Answer from the drawing. Dimensions are ordinates in mm from the lowest x, y and z of the part. Coordinates: 2 decimals unless noted, no trailing zeros. Order: outer loops, then holes, each group sorted by start corner. A loop starts at its lowest first (then second) coordinate and runs counter-clockwise, first axis right, second up. Notation, with made-up numbers: (44.5, -7.5) - (91.5, -7.5) arc R19 ccw to (91.5, -3.5) - close; hole circle Ø4 at (-14, 71). An arc over 180 degrees is marked (long way). Answer as a JSON object with one key per item and string values. Group by question number.
1) Section A-A (x = 45) is taken. Give the vertices of the cut face in (y, z), plus the area to 3 significant figures.
2) Each of these flat-tipped pins is pushed along its axis until it touches: P1, Ø5, axis at x = 49, y = 64.5, coming from the +Z side; P2, Ø4, axis at x = 49, z = 29.5, coming from the +Y side; P3, Ø5, axis at x = 15, z = 20, coming from the +Y side. Where does it stop, or does it pass through?
3) The mould has two halves that part along X. Classify the marked faces 1, 2 and 3: released by +X, released by -X, zero draft, split by the parting line, or undercut.
4) Section B-B (z = 50) is taken. Give the vertices of the cut face in (x, y), plus the area to 3 significant figures.
5) Find the intervals of material crossed by line 1 along Y through (x, z) = (15, 2.9); line 2 along Z through (x, y) = (45, 3.05); line 3 along X through (y, z) = (64, 7), in increasing order.
6) Section C-C (y = 65) is taken. Give the vertices of the cut face in (x, z), plus the area to 3 significant figures.
7) Section D-D (x = 22.5) is taken. Give the vertices of the cut face in (y, z), plus the area to 3 significant figures.
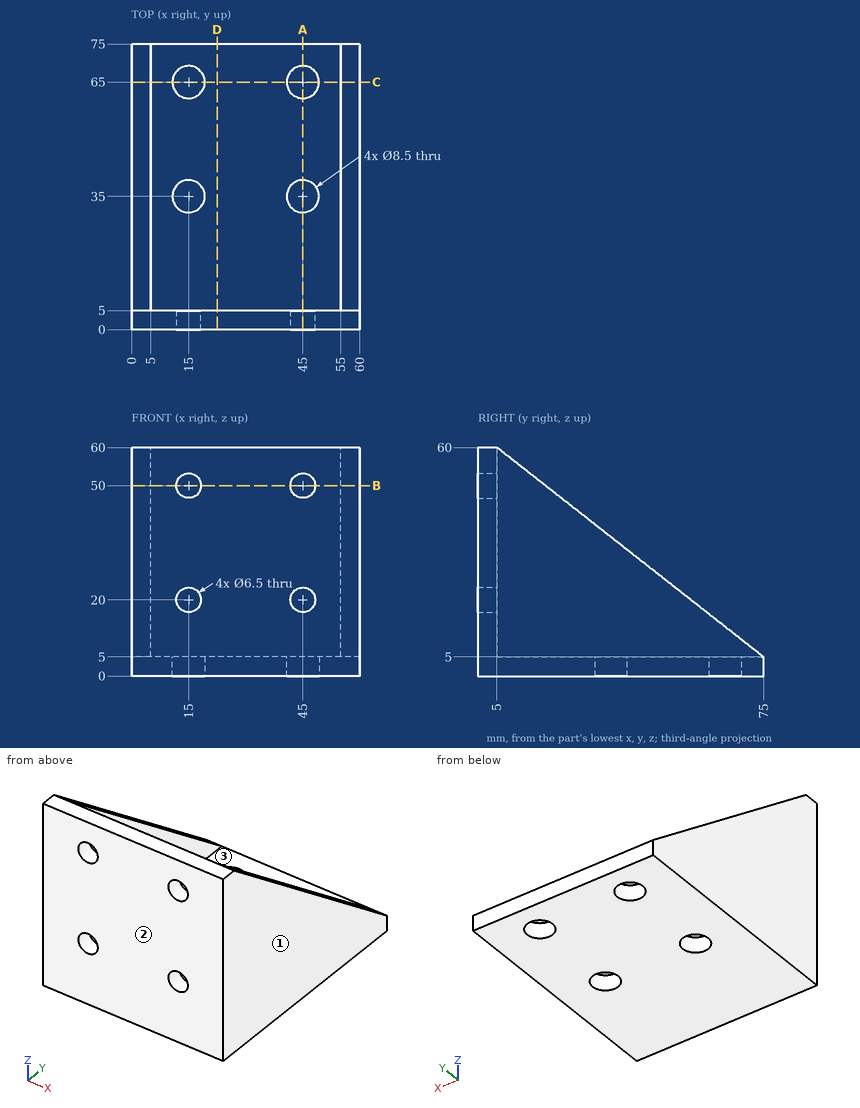
Report:
{
 "1": {"outline": "(0, 0) - (30.75, 0) - (30.75, 5) - (5, 5) - (5, 16.75) - (0, 16.75) - close; (0, 23.25) - (5, 23.25) - (5, 46.75) - (0, 46.75) - close; (0, 53.25) - (5, 53.25) - (5, 60) - (0, 60) - close; (39.25, 0) - (60.75, 0) - (60.75, 5) - (39.25, 5) - close; (69.25, 0) - (75, 0) - (75, 5) - (69.25, 5) - close", "area": "500 mm²"},
 "2": {"P1": "stops at z = 5", "P2": "stops at y = 5", "P3": "passes through"},
 "3": {"face 1": "released by +X", "face 2": "zero draft", "face 3": "undercut"},
 "4": {"outline": "(0, 0) - (11.75, 0) - (11.75, 5) - (5, 5) - (5, 17.73) - (0, 17.73) - close; (18.25, 0) - (41.75, 0) - (41.75, 5) - (18.25, 5) - close; (48.25, 0) - (60, 0) - (60, 17.73) - (55, 17.73) - (55, 5) - (48.25, 5) - close", "area": "362 mm²"},
 "5": {"line 1": "y = 0 to 30.75, 39.25 to 60.75, 69.25 to 75", "line 2": "z = 0 to 16.75, 23.25 to 46.75, 53.25 to 60", "line 3": "x = 0 to 5, 55 to 60"},
 "6": {"outline": "(0, 0) - (10.75, 0) - (10.75, 5) - (5, 5) - (5, 12.86) - (0, 12.86) - close; (19.25, 0) - (40.75, 0) - (40.75, 5) - (19.25, 5) - close; (49.25, 0) - (60, 0) - (60, 12.86) - (55, 12.86) - (55, 5) - (49.25, 5) - close", "area": "294 mm²"},
 "7": {"outline": "(0, 0) - (75, 0) - (75, 5) - (5, 5) - (5, 60) - (0, 60) - close", "area": "650 mm²"}
}
